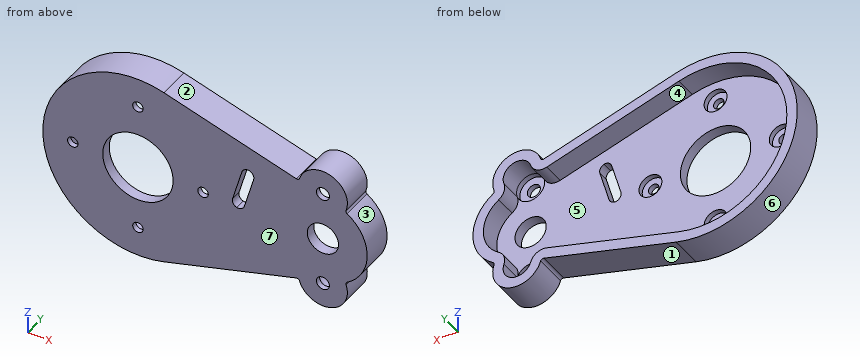
```python
from build123d import *

# Parameters (mm, degrees)
SKETCH1_W               = 175
SKETCH1_H               = 100
SKETCH1_R               = 6
SKETCH1_R_2             = 13.5
SKETCH1_R_3             = 2
SKETCH1_R_4             = 2.5
BOSS_EXTRUDE1_DEPTH     = 4
SKETCH3_W               = 175
SKETCH3_H               = 100
BOSS_EXTRUDE2_DEPTH     = 8.25
SKETCH6_R               = 5.4
CUT_EXTRUDE2_DEPTH      = 8.25
FILLET1_R               = 2.5
FILLET2_R               = 5
SKETCH2_R               = 4.4
SKETCH2_R_2             = 5.4
CUT_EXTRUDE1_DEPTH      = 2
CUT_EXTRUDE4_DEPTH      = 102.520010478
CUT_EXTRUDE4_DEPTH_BACK = 102.520010478
SKETCH7_OUTSIDE_W       = 217.386
SKETCH7_OUTSIDE_H       = 142.386


with BuildPart() as part:
    # Sketch1 → Boss-Extrude1 (new body)
    with BuildSketch(Plane(origin=(0, 0, 0), x_dir=(1, 0, 0), z_dir=(0, 1, 0))):
        Rectangle(SKETCH1_W, SKETCH1_H)
        with Locations(Location((35.5, 0, 0), (0, 0, 270))):
            Circle(SKETCH1_R, mode=Mode.SUBTRACT)
        with Locations(Location((-35.5, 0, 0), (0, 0, 270))):
            Circle(SKETCH1_R_2, mode=Mode.SUBTRACT)
        with Locations(Location((-60.5, 0, 0), (0, 0, 270))):
            Circle(SKETCH1_R_3, mode=Mode.SUBTRACT)
        with Locations(Location((-35.5, 25, 0), (0, 0, 270))):
            Circle(SKETCH1_R_3, mode=Mode.SUBTRACT)
        with Locations(Location((-10.5, 0, 0), (0, 0, 270))):
            Circle(SKETCH1_R_3, mode=Mode.SUBTRACT)
        with Locations(Location((-35.5, -25, 0), (0, 0, 270))):
            Circle(SKETCH1_R_3, mode=Mode.SUBTRACT)
        with Locations(Location((35.5, 18.5, 0), (0, 0, 270))):
            Circle(SKETCH1_R_4, mode=Mode.SUBTRACT)
        with Locations(Location((35.5, -18.5, 0), (0, 0, 90))):
            Circle(SKETCH1_R_4, mode=Mode.SUBTRACT)
        Polygon((4.517711304, -15.136418767), (0.159242352, 0.258507293), (4.681501882, 1.538807548), (9.039970835, -13.856118512), (9.584779454, -15.78048427), (5.062519924, -17.060784524), align=None, mode=Mode.SUBTRACT)
    extrude(amount=BOSS_EXTRUDE1_DEPTH)

    # Sketch3 → Boss-Extrude2 (add)
    with BuildSketch(Plane(origin=(0, 4, 0), x_dir=(1, 0, 0), z_dir=(0, 1, 0))):
        Rectangle(SKETCH3_W, SKETCH3_H)
        with BuildLine():
            Line((-26.573943662, 31.250208291), (39.070422535, 12.500083317))
            ThreePointArc((39.070422535, 12.500083317), (48.5, 0), (39.070422535, -12.500083317))
            Line((39.070422535, -12.500083317), (-26.573943662, -31.250208291))
            ThreePointArc((-26.573943662, -31.250208291), (-68, 0), (-26.573943662, 31.250208291))
        make_face(mode=Mode.SUBTRACT)
    extrude(amount=BOSS_EXTRUDE2_DEPTH)

    # Sketch6 → Cut-Extrude2 (cut)
    with BuildSketch(Plane(origin=(0, 12.25, 0), x_dir=(1, 0, 0), z_dir=(0, 1, 0))):
        with Locations((35.5, 18.5)):
            Circle(SKETCH6_R)
        with Locations((35.5, -18.5)):
            Circle(SKETCH6_R)
    extrude(amount=-CUT_EXTRUDE2_DEPTH, mode=Mode.SUBTRACT)

    # Fillet1
    # the kernel refuses this fillet: 2.5 mm, written as the material it adds along each edge
    with BuildSketch(Plane(origin=(9.584779454, 0, 15.78048427), x_dir=(-0.9621828787440704, 0, 0.2724043095323078), z_dir=(0, 1, 0)), Plane(origin=(5.062519924, 0, 17.060784524), x_dir=(-0.2724043095323173, 0, -0.9621828787440677), z_dir=(0, 1, 0)), Plane(origin=(4.681501882, 0, -1.538807548), x_dir=(0.2724043095323092, 0, 0.96218287874407), z_dir=(0, 1, 0))) as fillet1_piece_1:
        with BuildLine():
            CenterArc((FILLET1_R, -FILLET1_R), FILLET1_R, 90, 90)
            Line((0, -FILLET1_R), (0, 0))
            Line((0, 0), (FILLET1_R, 0))
        make_face()
    extrude(amount=4)
    with BuildSketch(Plane(origin=(0.159242352, 0, -0.258507293), x_dir=(0.2724043095323079, 0, 0.9621828787440704), z_dir=(0, 1, 0))) as fillet1_piece_2:
        with BuildLine():
            CenterArc((FILLET1_R, FILLET1_R), FILLET1_R, 180, 90)
            Line((0, FILLET1_R), (0, 0))
            Line((0, 0), (FILLET1_R, 0))
        make_face()
    extrude(amount=4)

    # Fillet2
    fillet2_edges = [part.edges().sort_by_distance(p)[0] for p in [
        (31.784909874, 8.125, 14.581058133),
        (36.584743308, 8.125, 13.210072594),
        (36.584743308, 8.125, -13.210072594),
        (31.784909874, 8.125, -14.581058133),
    ]]
    fillet(fillet2_edges, radius=FILLET2_R)

    # Sketch2 → Cut-Extrude1 (cut)
    with BuildSketch(Plane(origin=(0, 4, 0), x_dir=(1, 0, 0), z_dir=(0, 1, 0))):
        with Locations(Location((-35.5, 25, 0), (0, 0, 270))):
            Circle(SKETCH2_R)
        with Locations(Location((-10.5, 0, 0), (0, 0, 270))):
            Circle(SKETCH2_R)
        with Locations(Location((-35.5, -25, 0), (0, 0, 270))):
            Circle(SKETCH2_R)
        with Locations(Location((-60.5, 0, 0), (0, 0, 270))):
            Circle(SKETCH2_R)
        with Locations(Location((35.5, 18.5, 0), (0, 0, 270))):
            Circle(SKETCH2_R_2)
        with Locations(Location((35.5, -18.5, 0), (0, 0, 197.105868404))):
            Circle(SKETCH2_R_2)
    extrude(amount=-CUT_EXTRUDE1_DEPTH, mode=Mode.SUBTRACT)

    # Sketch7 outside → Cut-Extrude4 (cut, two sides: drawn at the far end of the back side and taken through both)
    with BuildSketch(Plane(origin=(0, 12.25, 0), x_dir=(1, 0, 0), z_dir=(0, 1, 0)).offset(-CUT_EXTRUDE4_DEPTH_BACK)):
        Rectangle(SKETCH7_OUTSIDE_W, SKETCH7_OUTSIDE_H)
        with BuildLine():
            Line((-25.475352113, -35.096387773), (25.285418022, -20.597492606))
            ThreePointArc((25.285418022, -20.597492606), (26.036864948, -20.680025145), (26.515828803, -21.264899257))
            ThreePointArc((26.515828803, -21.264899257), (38.426917352, -27.432701429), (44.378310133, -15.41202183))
            ThreePointArc((44.378310133, -15.41202183), (44.376580158, -14.760021946), (44.777099477, -14.245540541))
            ThreePointArc((44.777099477, -14.245540541), (52.5, 0), (44.777099477, 14.245540541))
            ThreePointArc((44.777099477, 14.245540541), (44.376580158, 14.760021946), (44.378310133, 15.41202183))
            ThreePointArc((44.378310133, 15.41202183), (38.426917352, 27.432701429), (26.515828803, 21.264899257))
            ThreePointArc((26.515828803, 21.264899257), (26.036864948, 20.680025145), (25.285418022, 20.597492606))
            Line((25.285418022, 20.597492606), (-25.475352113, 35.096387773))
            ThreePointArc((-25.475352113, 35.096387773), (-72, 0), (-25.475352113, -35.096387773))
        make_face(mode=Mode.SUBTRACT)
    extrude(amount=CUT_EXTRUDE4_DEPTH + CUT_EXTRUDE4_DEPTH_BACK, mode=Mode.SUBTRACT)


solid = part.part
```
Work out the finished part from the listing and answer in its coordinate system (mm). Face numbers are marked on the shaded views. A direction names the side the tool comes from. Give positions to 0.01 mm unless a question says otherwise; leave off trailing zeros. Loops run counter-clockwise (first coordinate to the right, second up) from the corner with the lowest first, then second, coordinate; pieces in that order, holes last. Notation, with made-up numbers: (30.5, -33.5) -> (43.5, -33.5) arc R3 cw to (43.5, -29.5) -> close; hole circle Ø6 at (76, 64). An arc over 180 degrees is marked (long way). Put each result on its own line as item: value. Start each with the question number.
Item 1: The part is cut by section C-C (x = -35.5). Give the vertices of the cut face in (y, z), then the cut area to 3 significant figures.
Item 2: The part is cut by section B-B (x = -60.5). Give the vertices of the cut face in (y, z), then the cut area to 3 significant figures.
Item 3: Find the intervals of material crossed by L1, parallel to X at y = 6.25, z = 0; L2, parallel to X at y = 3.5, z = 0; L3, parallel to Y at x = -12, z = -25.5, in increasing order. Write a range as [from, to].
Item 4: Each of these flat-tipped pins is pushed along its axis until it touches: P1, Ø1.5, axis at x = 0.5, y = 10, coming from the -Z side; P2, Ø3, axis at x = -35.5, z = -25, coming from the -Y side; P3, Ø4.5, axis at x = -37.5, z = 24.5, coming from the +Y side; P4, Ø2, axis at x = -15, y = 7.5, coming from the +Z side. Where does it stop, or does it pass through?
Item 5: The part is cut by section D-D (x = -10.5). Give the vertices of the cut face in (y, z), then the cut area to 3 significant figures.
Item 6: The part is cut by section A-A (x = 35.5). Give the vertices of the cut face in (y, z), then the cut area to 3 significant figures.
Item 7: Which of the six approach directions +Z, -Z, +X, -X, +Y, -Y give full straight-line access (tool end or side, diameter ignored) to the marked faces 1, 2, 3 and 4?
Item 8: The mould has two halves that part along Z. Classify the marked faces 5, 6 and 7: released by +Z, released by -Z, zero draft, split by the parting line, or undercut.
Answers below:
1. outline: (0, -36.5) -> (12.25, -36.5) -> (12.25, -32.5) -> (4, -32.5) -> (4, -29.4) -> (2, -29.4) -> (2, -27) -> (0, -27) -> close; (0, -23) -> (2, -23) -> (2, -20.6) -> (4, -20.6) -> (4, -13.5) -> (0, -13.5) -> close; (0, 13.5) -> (4, 13.5) -> (4, 20.6) -> (2, 20.6) -> (2, 23) -> (0, 23) -> close; (0, 27) -> (2, 27) -> (2, 29.4) -> (4, 29.4) -> (4, 32.5) -> (12.25, 32.5) -> (12.25, 36.5) -> (0, 36.5) -> close
1. area: 199 mm2
2. outline: (0, -26.59) -> (12.25, -26.59) -> (12.25, -20.77) -> (4, -20.77) -> (4, -4.4) -> (2, -4.4) -> (2, -2) -> (0, -2) -> close; (0, 2) -> (2, 2) -> (2, 4.4) -> (4, 4.4) -> (4, 20.77) -> (12.25, 20.77) -> (12.25, 26.59) -> (0, 26.59) -> close
2. area: 283 mm2
3. L1: [-72, -68], [48.5, 52.5]
3. L2: [-72, -64.9], [-56.1, -49], [-22, -14.9], [-6.1, 1.22], [4.92, 29.5], [41.5, 52.5]
3. L3: [0, 4]
4. P1: z = -27.89
4. P2: through
4. P3: y = 2
4. P4: z = 32.39
5. outline: (0, -30.82) -> (12.25, -30.82) -> (12.25, -26.66) -> (4, -26.66) -> (4, -4.4) -> (2, -4.4) -> (2, -2) -> (0, -2) -> close; (0, 2) -> (2, 2) -> (2, 4.4) -> (4, 4.4) -> (4, 26.66) -> (12.25, 26.66) -> (12.25, 30.82) -> (0, 30.82) -> close
5. area: 290 mm2
6. outline: (0, -27.9) -> (12.25, -27.9) -> (12.25, -23.9) -> (2, -23.9) -> (2, -21) -> (0, -21) -> close; (0, -16) -> (2, -16) -> (2, -13.1) -> (4, -13.1) -> (4, -6) -> (0, -6) -> close; (0, 6) -> (4, 6) -> (4, 13.1) -> (2, 13.1) -> (2, 16) -> (0, 16) -> close; (0, 21) -> (2, 21) -> (2, 23.9) -> (12.25, 23.9) -> (12.25, 27.9) -> (0, 27.9) -> close
6. area: 178 mm2
7. face 1: -Z, +Y, -Y
7. face 2: +Z, +Y, -Y
7. face 3: +X, +Y, -Y
7. face 4: +Y
8. face 5: undercut
8. face 6: split by the parting line
8. face 7: zero draft
